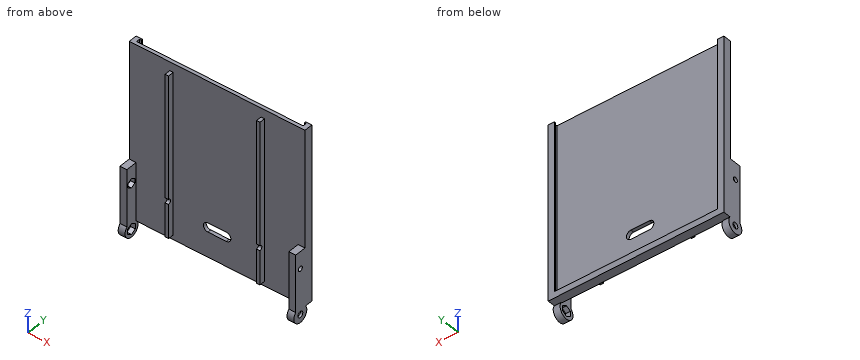
```python
from build123d import *

# Parameters (mm, degrees)
CROQUIS_PLACA_W                      = 153.8
CROQUIS_PLACA_H                      = 153.8
PLACA_DEPTH                          = 3
CROQUIS_BORDE_IZQ_W                  = 4
CROQUIS_BORDE_IZQ_H                  = 153.8
BORDE_IZQ_DEPTH                      = 3.2
CROQUIS_BORDE_DER_W                  = 4
CROQUIS_BORDE_DER_H                  = 153.8
BORDE_DER_DEPTH                      = 3.2
CROQUIS_BORDE_TRAS_W                 = 145.8
CROQUIS_BORDE_TRAS_H                 = 4
BORDE_TRAS_DEPTH                     = 3.2
CROQUIS_CEJA_IZQ_W                   = 5.5
CROQUIS_CEJA_IZQ_H                   = 153.8
CEJA_IZQ_DEPTH                       = 1.2
CROQUIS_CEJA_DER_W                   = 5.5
CROQUIS_CEJA_DER_H                   = 153.8
CEJA_DER_DEPTH                       = 1.2
CROQUIS_CEJA_TRAS_W                  = 148.3
CROQUIS_CEJA_TRAS_H                  = 5.5
CEJA_TRAS_DEPTH                      = 1.2
PASO_CABLE_DEPTH                     = 176.977867927
PASO_CABLE_DEPTH_BACK                = 176.977867927
CROQUIS_REFUERZOS_W                  = 3
CROQUIS_REFUERZOS_H                  = 142
REFUERZOS_DEPTH                      = 5
CROQUIS_COSTILLA_DER_W               = 55
CROQUIS_COSTILLA_DER_H               = 10
COSTILLA_DER_DEPTH                   = 6
CROQUIS_BUJE_DER_R                   = 7
BUJE_DER_DEPTH                       = 6
CROQUIS_COSTILLA_IZQ_W               = 55
CROQUIS_COSTILLA_IZQ_H               = 10
COSTILLA_IZQ_DEPTH                   = 6
BUJE_IZQ_START                       = -6
CROQUIS_BUJE_IZQ_R                   = 7
BUJE_IZQ_DEPTH                       = 6
AGUJEROS_PIVOTE_Y_BLOQUEO_DEPTH      = 176.977867927
AGUJEROS_PIVOTE_Y_BLOQUEO_DEPTH_BACK = 176.977867927
CROQUIS_AGUJEROS_EJE_R               = 2.65
CROQUIS_AGUJEROS_EJE_R_2             = 2.15
TUERCA_M5_DER_DEPTH                  = 4
TUERCAS_M5_M4_IZQ_DEPTH              = 4


with BuildPart() as part:
    # Croquis_placa → Placa (new body)
    with BuildSketch(Plane(origin=(0, 5, 0), x_dir=(1, 0, 0), z_dir=(0, 1, 0))):
        with Locations((0, -80.9)):
            Rectangle(CROQUIS_PLACA_W, CROQUIS_PLACA_H)
    extrude(amount=PLACA_DEPTH)

    # Croquis_Borde_izq → Borde_izq (add)
    with BuildSketch(Plane(origin=(0, 8, 0), x_dir=(1, 0, 0), z_dir=(0, 1, 0))):
        with Locations((-74.9, -80.9)):
            Rectangle(CROQUIS_BORDE_IZQ_W, CROQUIS_BORDE_IZQ_H)
    extrude(amount=BORDE_IZQ_DEPTH)

    # Croquis_Borde_der → Borde_der (add)
    with BuildSketch(Plane(origin=(0, 8, 0), x_dir=(1, 0, 0), z_dir=(0, 1, 0))):
        with Locations((74.9, -80.9)):
            Rectangle(CROQUIS_BORDE_DER_W, CROQUIS_BORDE_DER_H)
    extrude(amount=BORDE_DER_DEPTH)

    # Croquis_Borde_tras → Borde_tras (add)
    with BuildSketch(Plane(origin=(0, 8, 0), x_dir=(1, 0, 0), z_dir=(0, 1, 0))):
        with Locations((0, -6)):
            Rectangle(CROQUIS_BORDE_TRAS_W, CROQUIS_BORDE_TRAS_H)
    extrude(amount=BORDE_TRAS_DEPTH)

    # Croquis_Ceja_izq → Ceja_izq (add)
    with BuildSketch(Plane(origin=(0, 11.2, 0), x_dir=(1, 0, 0), z_dir=(0, 1, 0))):
        with Locations((-74.15, -80.9)):
            Rectangle(CROQUIS_CEJA_IZQ_W, CROQUIS_CEJA_IZQ_H)
    extrude(amount=CEJA_IZQ_DEPTH)

    # Croquis_Ceja_der → Ceja_der (add)
    with BuildSketch(Plane(origin=(0, 11.2, 0), x_dir=(1, 0, 0), z_dir=(0, 1, 0))):
        with Locations((74.15, -80.9)):
            Rectangle(CROQUIS_CEJA_DER_W, CROQUIS_CEJA_DER_H)
    extrude(amount=CEJA_DER_DEPTH)

    # Croquis_Ceja_tras → Ceja_tras (add)
    with BuildSketch(Plane(origin=(0, 11.2, 0), x_dir=(1, 0, 0), z_dir=(0, 1, 0))):
        with Locations((0, -6.75)):
            Rectangle(CROQUIS_CEJA_TRAS_W, CROQUIS_CEJA_TRAS_H)
    extrude(amount=CEJA_TRAS_DEPTH)

    # Croquis_cable → Paso_cable (cut, two sides: drawn at the far end of the back side and taken through both)
    with BuildSketch(Plane(origin=(0, 0, 0), x_dir=(1, 0, 0), z_dir=(0, 1, 0)).offset(-PASO_CABLE_DEPTH_BACK)):
        with BuildLine():
            Line((-8, -26), (8, -26))
            ThreePointArc((8, -26), (12, -30), (8, -34))
            Line((8, -34), (-8, -34))
            ThreePointArc((-8, -34), (-12, -30), (-8, -26))
        make_face()
    extrude(amount=PASO_CABLE_DEPTH + PASO_CABLE_DEPTH_BACK, mode=Mode.SUBTRACT)

    # Croquis_refuerzos → Refuerzos (add)
    with BuildSketch(Plane(origin=(0, 5, 0), x_dir=(1, 0, 0), z_dir=(0, 1, 0))):
        with Locations((-40, -79)):
            Rectangle(CROQUIS_REFUERZOS_W, CROQUIS_REFUERZOS_H)
        with Locations((40, -79)):
            Rectangle(CROQUIS_REFUERZOS_W, CROQUIS_REFUERZOS_H)
    extrude(amount=-REFUERZOS_DEPTH)

    # Croquis_costilla_der → Costilla_der (add)
    with BuildSketch(Plane(origin=(70.9, 0, 0), x_dir=(0, 0, -1), z_dir=(1, 0, 0))):
        with Locations((-27.5, 0)):
            Rectangle(CROQUIS_COSTILLA_DER_W, CROQUIS_COSTILLA_DER_H)
    extrude(amount=COSTILLA_DER_DEPTH)

    # Croquis_buje_der → Buje_der (add)
    with BuildSketch(Plane(origin=(70.9, 0, 0), x_dir=(0, 0, -1), z_dir=(1, 0, 0))):
        Circle(CROQUIS_BUJE_DER_R)
    extrude(amount=BUJE_DER_DEPTH)

    # Croquis_costilla_izq → Costilla_izq (add)
    with BuildSketch(Plane(origin=(-70.9, 0, 0), x_dir=(0, 0, -1), z_dir=(1, 0, 0))):
        with Locations((-27.5, 0)):
            Rectangle(CROQUIS_COSTILLA_IZQ_W, CROQUIS_COSTILLA_IZQ_H)
    extrude(amount=-COSTILLA_IZQ_DEPTH)

    # Croquis_buje_izq → Buje_izq (add)
    with BuildSketch(Plane(origin=(-70.9, 0, 0), x_dir=(0, 0, -1), z_dir=(1, 0, 0)).offset(BUJE_IZQ_START)):
        Circle(CROQUIS_BUJE_IZQ_R)
    extrude(amount=BUJE_IZQ_DEPTH)

    # Croquis_agujeros_eje → Agujeros_pivote_y_bloqueo (cut, two sides: drawn at the far end of the back side and taken through both)
    with BuildSketch(Plane(origin=(0, 0, 0), x_dir=(0, 0, -1), z_dir=(1, 0, 0)).offset(-AGUJEROS_PIVOTE_Y_BLOQUEO_DEPTH_BACK)):
        with Locations(Location((0, 0, 0), (0, 0, 180))):
            Circle(CROQUIS_AGUJEROS_EJE_R)
        with Locations(Location((-40, 0, 0), (0, 0, 180))):
            Circle(CROQUIS_AGUJEROS_EJE_R_2)
    extrude(amount=AGUJEROS_PIVOTE_Y_BLOQUEO_DEPTH + AGUJEROS_PIVOTE_Y_BLOQUEO_DEPTH_BACK, mode=Mode.SUBTRACT)

    # Croquis_tuerca_M5_der → Tuerca_M5_der (cut)
    with BuildSketch(Plane(origin=(70.9, 0, 0), x_dir=(0, 0, -1), z_dir=(1, 0, 0))):
        Polygon((4.734272207, 0), (2.367136104, 4.1), (-2.367136104, 4.1), (-4.734272207, 0), (-2.367136104, -4.1), (2.367136104, -4.1), align=None)
    extrude(amount=TUERCA_M5_DER_DEPTH, mode=Mode.SUBTRACT)

    # Croquis_tuercas_izq → Tuercas_M5_M4_izq (cut)
    with BuildSketch(Plane(origin=(-70.9, 0, 0), x_dir=(0, 0, -1), z_dir=(1, 0, 0))):
        Polygon((4.734272207, 0), (2.367136104, 4.1), (-2.367136104, 4.1), (-4.734272207, 0), (-2.367136104, -4.1), (2.367136104, -4.1), align=None)
        Polygon((-35.843078062, 0), (-37.921539031, 3.6), (-42.078460969, 3.6), (-44.156921938, 0), (-42.078460969, -3.6), (-37.921539031, -3.6), align=None)
    extrude(amount=-TUERCAS_M5_M4_IZQ_DEPTH, mode=Mode.SUBTRACT)


solid = part.part
```
Can you work these out from the model? Positions are in its coordinate system, mm. Give positions to 0.01 mm unless a question says otherwise; leave off trailing zeros. Order: outer loops, then holes, each group sorted by start corner. A loop starts at its lowest first (then second) coordinate and runs counter-clockwise, first axis right, second up. Notation, with made-up numbers: M 45,50.5 L 82,50.5 A28 cw 82,78.5 Z; hole C 27,44 d9. An arc over 180 degrees is marked long. One line per item, written item: value.
1) I want a section at C-C, the plane x = 45. List the corners of the cut face in (y, z) for me.
Answer sheet:
outline: M 5,4 L 12.4,4 L 12.4,9.5 L 11.2,9.5 L 11.2,8 L 8,8 L 8,157.8 L 5,157.8 Z
2) I want a section at A-A, the plane z = 30. List the corners of the cut face in (x, y) for me.
Answer sheet:
outline: M -76.9,-5 L -70.9,-5 L -70.9,5 L -41.5,5 L -41.5,0 L -38.5,0 L -38.5,5 L -12,5 L -12,8 L -72.9,8 L -72.9,11.2 L -71.4,11.2 L -71.4,12.4 L -76.9,12.4 Z; M 12,5 L 38.5,5 L 38.5,0 L 41.5,0 L 41.5,5 L 70.9,5 L 70.9,-5 L 76.9,-5 L 76.9,12.4 L 71.4,12.4 L 71.4,11.2 L 72.9,11.2 L 72.9,8 L 12,8 Z
3) For P1, Ø3, axis at x = -72, z = 39.5, coming from the -Y side; P2, Ø3, axis at x = -75, y = 0.5, coming from the +Z side; P3, Ø10, axis at x = 12.5, y = -2, coming from the +Z side; P4, Ø4.5, axis at x = 72, z = 0, coming from the +Y side, each with a flat end and sliding along its axis, tell me the tip position at first contact or that it passes through.
Answer sheet:
P1: stops at y = -5
P2: stops at z = 55
P3: passes through
P4: stops at y = 7
4) I want a section at B-B, the plane z = 0. List the corners of the cut face in (x, y) for me, plus the area to 3 significant figures.
Answer sheet:
outline: M -76.9,-7 L -70.9,-7 L -70.9,-4.1 L -74.9,-4.1 L -74.9,-2.65 L -76.9,-2.65 Z; M -76.9,2.65 L -74.9,2.65 L -74.9,4.1 L -70.9,4.1 L -70.9,7 L -76.9,7 Z; M 70.9,-7 L 76.9,-7 L 76.9,-2.65 L 74.9,-2.65 L 74.9,-4.1 L 70.9,-4.1 Z; M 70.9,4.1 L 74.9,4.1 L 74.9,2.65 L 76.9,2.65 L 76.9,7 L 70.9,7 Z
area: 81.2 mm^2
5) I want a section at D-D, the plane z = 60.5. List the corners of the cut face in (x, y) for me.
Answer sheet:
outline: M -76.9,5 L -41.5,5 L -41.5,0 L -38.5,0 L -38.5,5 L 38.5,5 L 38.5,0 L 41.5,0 L 41.5,5 L 76.9,5 L 76.9,12.4 L 71.4,12.4 L 71.4,11.2 L 72.9,11.2 L 72.9,8 L -72.9,8 L -72.9,11.2 L -71.4,11.2 L -71.4,12.4 L -76.9,12.4 Z
6) Please list where these lines run through material, in increasing order: line 1 along X through (y, z) = (4.75, 119); line 2 along Y through (x, z) = (-75.4, 0); line 3 along Y through (x, z) = (-75.5, 40).
Answer sheet:
line 1: x = -41.5 to -38.5, 38.5 to 41.5
line 2: y = -7 to -2.65, 2.65 to 7
line 3: y = -5 to -2.15, 2.15 to 12.4
